Autodesk Inventor part; units mm, degrees
ref_plane "YZ Plane" through (0, 0, 0) normal (1, 0, 0) x (0, 1, 0)
ref_plane "XZ Plane" through (0, 0, 0) normal (0, 1, 0) x (-1, 0, 0)
ref_plane "XY Plane" through (0, 0, 0) normal (0, 0, 1) x (1, 0, 0)
sketch "Sketch1" plane through (0, 0, 0) normal (0, 1, 0) x (-1, 0, 0)
  line L0 (-9.3834, 9.4925) -> (22.3666, 9.4925)
  line L1 (22.3666, 9.4925) -> (22.3666, -47.6575)
  line L2 (22.3666, -47.6575) -> (-9.3834, -47.6575)
  line L3 (-9.3834, -47.6575) -> (-9.3834, 9.4925)
  point P0 (0, 0)
  dimension "d0" = 31.75
  dimension "d1" = 57.15
extrude "Extrusion1" add sketch "Sketch1" along normal blind 25.4
sketch "Sketch2" plane through (0, 25.4, 0) normal (0, 1, 0) x (1, 0, 0)
  point P0 (0, 0)
sketch "Sketch3" plane through (0, 25.4, 0) normal (0, 1, 0) x (1, 0, 0)
  line L0 (-22.3666, -9.4925) -> (9.3834, -9.4925) construction
  line L1 (-22.3666, -9.4925) -> (-9.6666, -9.4925) construction
  line L2 (9.3834, -9.4925) -> (-3.3166, -9.4925) construction
  line L3 (-9.6666, -9.4925) -> (-3.3166, -9.4925) construction
  line L4 (-3.3166, -9.4925) -> (-3.3166, 22.2575)
  line L5 (-3.3166, 22.2575) -> (-9.6666, 22.2575)
  line L6 (-9.6666, 22.2575) -> (-9.6666, -9.4925)
  line L7 (-9.6666, -9.4925) -> (-3.3166, -9.4925)
  point P0 (0, 0)
  dimension "d4" = 12.7
  dimension "d5" = 12.7
  dimension "d6" = 31.75
extrude "Extrusion2" cut sketch "Sketch3" against normal blind 25.4
sketch "Sketch4" plane through (0, 25.4, 0) normal (0, 1, 0) x (1, 0, 0)
  line L0 (9.3834, 47.6575) -> (9.3834, -9.4925)
  line L1 (-22.3666, 47.6575) -> (9.3834, 47.6575)
  line L2 (9.3834, 47.6575) -> (9.3834, 34.9575)
  line L3 (9.3834, 34.9575) -> (-22.3666, 34.9575)
  line L4 (-22.3666, 34.9575) -> (-22.3666, 47.6575)
  point P0 (0, 0)
  dimension "d9" = 12.7
extrude "Extrusion3" add sketch "Sketch4" along normal blind 12.7
sketch "Sketch5" plane through (0, 38.1, 0) normal (0, 1, 0) x (1, 0, 0)
  line L0 (9.3834, 34.9575) -> (-22.3666, 34.9575)
  line L1 (-22.3666, 47.6575) -> (9.3834, 47.6575)
  line L2 (9.3834, 34.9575) -> (3.0334, 34.9575)
  line L3 (3.0334, 34.9575) -> (3.0334, 47.6575)
  line L4 (3.0334, 47.6575) -> (9.3834, 47.6575)
  line L5 (9.3834, 47.6575) -> (9.3834, 34.9575)
  line L6 (-22.3666, 47.6575) -> (-16.0166, 47.6575)
  line L7 (-16.0166, 47.6575) -> (-16.0166, 34.9575)
  line L8 (-16.0166, 34.9575) -> (-22.3666, 34.9575)
  line L9 (-22.3666, 34.9575) -> (-22.3666, 47.6575)
  point P0 (0, 0)
  dimension "d12" = 6.35
  dimension "d13" = 6.35
extrude "Extrusion4" add sketch "Sketch5" along normal blind 6.35 contours L0 L3 L1 L5 | L0 L9 L1 L7
properties part number "Unit 7.1"
The listing builds one solid part. Answer for the finished solid, in the listing's coordinates (mm). A direction names the side the tool comes from. Coordinates: 2 decimals unless noted, no trailing zeros. Loops run counter-clockwise (first coordinate to the right, second up) from the corner with the lowest first, then second, coordinate; pieces in that order, holes last. Notation, with made-up numbers: (12.25, 79) - (37.25, 79) arc R17 cw to (37.25, 83) - close; hole circle Ø10 at (-35.75, -24). An arc over 180 degrees is marked (long way). Use a Markdown table: item, result. Add a question column.
1) Given pin 1 (9.5 mm diameter, centred on x = -10.5, y = 38, fed in from +Z); pin 2 (6 mm diameter, centred on x = -13, z = -4.5, fed in from +Y); pin 3 (10 mm diameter, centred on x = -2, z = -39, fed in from +Y), each flat-ended and moving along its own axis, determine where each tip first touches the part or whether it passes through.
2) For faces 1 (the flat face through (-3, 25.4, -12)), 2 (the flat face through (-16.017, 41, -41)), 3 (the flat face through (-9.667, 13, -7)), determine the directions among +Z, -Z, +X, -X, +Y, -Y from which every point of the face is accessible in a straight line to the end or side of a thin tool.
3) The part is cut by section B-B, the plane z = -9. Give the vertices of the cut face in (x, y).
4) The part is cut by section C-C, the plane x = 4.5. Give the vertices of the cut face in (y, z).
5) The part is cut by section A-A, the plane y = 41.5. Give the vertices of the cut face in (x, z).
6) The part is cut by section D-D, the plane y = 24.5. Give the vertices of the cut face in (x, z).
7) Find the intervals of material crossed by line 1 (X direction, y = 7.5, z = -17); line 2 (Y direction, x = -16.5, z = 0); line 3 (Y direction, x = -8, z = -38), in increasing order.
Here are the results:
| question | item | result |
|---|---|---|
| 1 | pin 1 | stops at z = -34.96 |
| 1 | pin 2 | stops at y = 25.4 |
| 1 | pin 3 | stops at y = 38.1 |
| 2 | face 1 | +Z, +X, -X, +Y |
| 2 | face 2 | +Z, -Z, +Y |
| 2 | face 3 | +Z, +Y, -Y |
| 3 | outline | (-22.37, 0) - (-9.67, 0) - (-9.67, 25.4) - (-22.37, 25.4) - close; (-3.32, 0) - (9.38, 0) - (9.38, 25.4) - (-3.32, 25.4) - close |
| 4 | outline | (0, -47.66) - (44.45, -47.66) - (44.45, -34.96) - (25.4, -34.96) - (25.4, 9.49) - (0, 9.49) - close |
| 5 | outline | (-22.37, -47.66) - (-16.02, -47.66) - (-16.02, -34.96) - (-22.37, -34.96) - close; (3.03, -47.66) - (9.38, -47.66) - (9.38, -34.96) - (3.03, -34.96) - close |
| 6 | outline | (-22.37, -47.66) - (9.38, -47.66) - (9.38, 9.49) - (-3.32, 9.49) - (-3.32, -22.26) - (-9.67, -22.26) - (-9.67, 9.49) - (-22.37, 9.49) - close |
| 7 | line 1 | x = -22.37 to -9.67, -3.32 to 9.38 |
| 7 | line 2 | y = 0 to 25.4 |
| 7 | line 3 | y = 0 to 38.1 |
